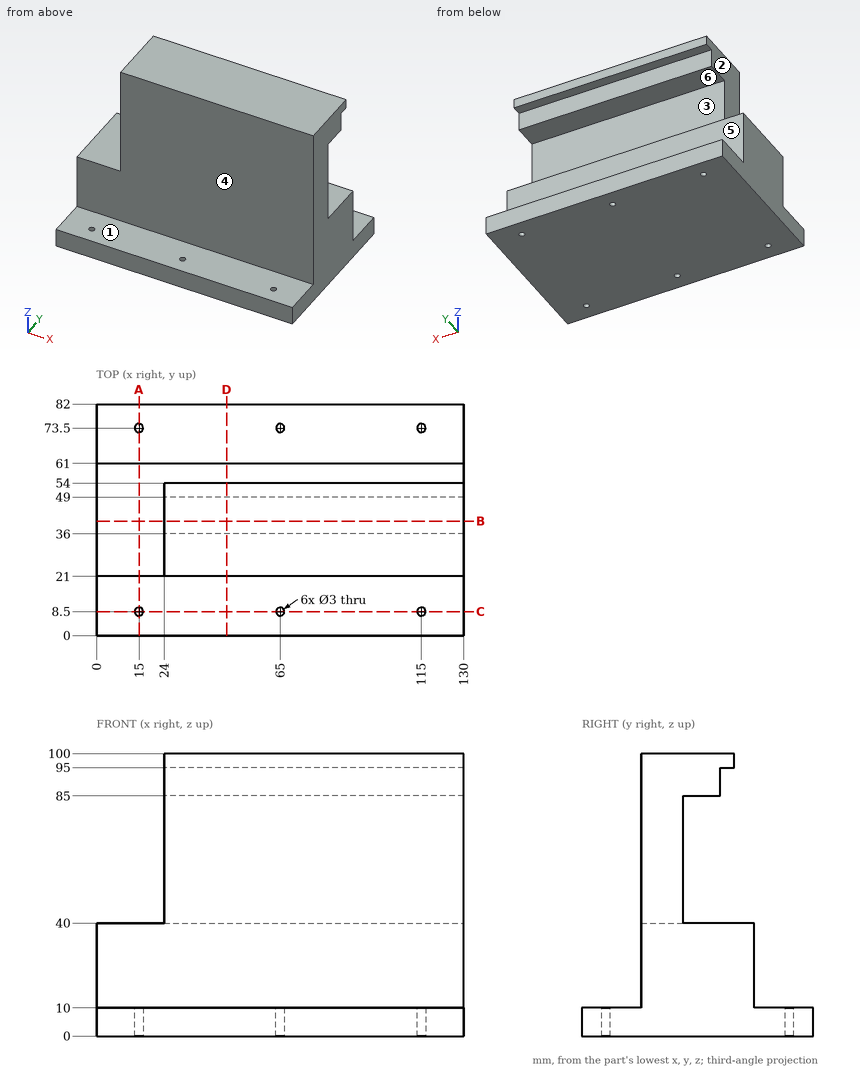
Can you work these out from the drawing? Everything is in mm from the part's minimum corner. A direction names the side the tool comes from. Coordinates: 2 decimals unless noted, no trailing zeros. Loops run counter-clockwise (first coordinate to the right, second up) from the corner with the lowest first, then second, coordinate; pieces in that order, holes last. Notation, with made-up numbers: (81.5, 24.25) -> (86.5, 24.25) arc R13 cw to (86.5, 48.25) -> close; hole circle Ø1 at (-38, 76). An arc over 180 degrees is marked (long way). Return JSON: item names as keys, results as strings.
1) Will these pins go through, and if not, where does the flat tip stop? pin 1 (15 mm diameter, centred on x = 53.5, z = 29, fed in from +Y); pin 2 (3.5 mm diameter, centred on x = 115, y = 8.5, fed in from +Z); pin 3 (2 mm diameter, centred on x = 24, z = 49.5, fed in from -Y); pin 4 (1.8 mm diameter, centred on x = 15, y = 8.5, fed in from -Z).
Results below:
{"pin 1": "y = 61", "pin 2": "z = 10", "pin 3": "y = 21", "pin 4": "through"}
2) I need wall thicknesses on line 1 (X direction, y = 73.5, z = 5); line 2 (Y direction, x = 15, z = 8); line 3 (Z direction, x = 55.5, y = 13). Which ranges of each line are inside material? Lowest first, please. Write a range as from..to.
Results below:
{"line 1": "0..13.5, 16.5..63.5, 66.5..113.5, 116.5..130", "line 2": "0..7, 10..72, 75..82", "line 3": "0..10"}
3) If we section it at D-D, the plane x = 46: Write out the boundary of the cut face in (y, z).
Results below:
{"outline": "(0, 0) -> (82, 0) -> (82, 10) -> (61, 10) -> (61, 40) -> (36, 40) -> (36, 85) -> (49, 85) -> (49, 95) -> (54, 95) -> (54, 100) -> (21, 100) -> (21, 10) -> (0, 10) -> close"}
4) For the marked faces 4, 5 and 6, which set-ups out of +Z, -Z, +X, -X, +Y, -Y let a thin tool reach every point of the face, with its end or its side?
Results below:
{"face 4": "+Z, +X, -X, -Y", "face 5": "+Z, +X, -X, +Y", "face 6": "+X, -X, +Y"}
5) If we section it at B-B, the plane y = 40.5: Write out the boundary of the cut face in (x, z), then the cut area to 3 significant figures.
Results below:
{"outline": "(0, 0) -> (130, 0) -> (130, 40) -> (0, 40) -> close; (24, 85) -> (130, 85) -> (130, 100) -> (24, 100) -> close", "area": "6,790 mm²"}
6) If we section it at A-A, the plane x = 15: Write out the boundary of the cut face in (y, z), then the cut area to 3 significant figures.
Results below:
{"outline": "(0, 0) -> (7, 0) -> (7, 10) -> (0, 10) -> close; (10, 0) -> (72, 0) -> (72, 10) -> (61, 10) -> (61, 40) -> (21, 40) -> (21, 10) -> (10, 10) -> close; (75, 0) -> (82, 0) -> (82, 10) -> (75, 10) -> close", "area": "1,960 mm²"}
7) Thinking about a two-plate mould opening in Z: for the marked faces 1, 2 and 3, which applies, +Z half, -Z half, draft (parallel to the pull), parting line (faces both ways), or undercut?
Results below:
{"face 1": "+Z half", "face 2": "draft", "face 3": "undercut"}
8) If we section it at C-C, the plane y = 8.5: Write out the boundary of the cut face in (x, z).
Results below:
{"outline": "(0, 0) -> (13.5, 0) -> (13.5, 10) -> (0, 10) -> close; (16.5, 0) -> (63.5, 0) -> (63.5, 10) -> (16.5, 10) -> close; (66.5, 0) -> (113.5, 0) -> (113.5, 10) -> (66.5, 10) -> close; (116.5, 0) -> (130, 0) -> (130, 10) -> (116.5, 10) -> close"}
